Build history of the part. All positions in model axes, mm. Face numbers are marked on the shaded views. Round coordinates to 2 decimals unless told otherwise and drop trailing zeros. Loops run counter-clockwise (first coordinate to the right, second up) from the corner with the lowest first, then second, coordinate; pieces in that order, holes last.
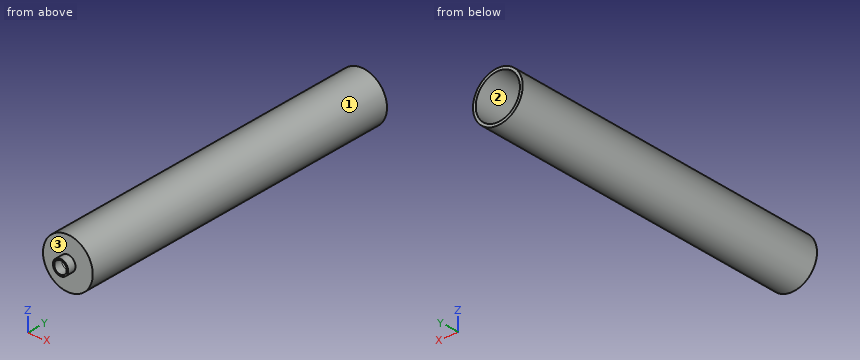
from build123d import *

# Parameters (mm, degrees)
F0_R     = 2.75
F0_R_2   = 2.25
F1_DEPTH = 3
F2_R     = 9
F3_DEPTH = 120
F4_T     = 1
F5_DEPTH = 25


# Not quite as in the source:
# - a shell that OpenCascade refuses in one call is made with other operations: the cavity is built on its own and cut out


with BuildPart() as f1:
    # F0 (on Front) → F1 (new body)
    with BuildSketch(Plane.XZ):
        Circle(F0_R)
        Circle(F0_R_2, mode=Mode.SUBTRACT)
    extrude(amount=F1_DEPTH)

    # F2 (on face) → F3 (join)
    with BuildSketch(Plane(origin=(0, 0, 0), x_dir=(-1, 0, 0), z_dir=(0, 1, 0))):
        Circle(F2_R)
    extrude(amount=F3_DEPTH)

    # F4: shell of thickness 1, made by hand


with BuildPart() as f4_core1:
    # F4_t2: copy of F1
    add(f1.part)

    # the walls: a layer under each face that stays
    f4_faces = [f4_core1.faces().sort_by_distance(p)[0] for p in [
        (9, 60, 0),
        (6, 0, -6),
        (-2.75, -1.5, 0),
        (-1.8333333333, -3, -1.8333333333),
        (-2.25, -1.5, 0),
        (0, 0, 0),
    ]]
    thicken(f4_faces, amount=-F4_T, mode=Mode.SUBTRACT)

    # F4_s3 → F4_t4 (revolve, cut)
    with BuildSketch(Plane.XY):
        Polygon((2.76, -0.01), (2.75, 1), (1.75, 1), (1.75, 0), align=None)
    revolve(axis=Axis((0, 0, 0), (0, -1, 0)), mode=Mode.SUBTRACT)

    # F4_s5 → F4_t6 (revolve, cut)
    with BuildSketch(Plane.XY):
        Polygon((2.24, -0.01), (3.25, 0), (3.25, 1), (2.25, 1), align=None)
    revolve(axis=Axis((0, 0, 0), (0, -1, 0)), mode=Mode.SUBTRACT)


with BuildPart() as f1_1:
    add(f1.part)

    # what is left inside the walls is the cavity
    f4_cavity = [f4_core1.part.solids().sort_by_distance(p)[0] for p in [
        (7.99, 80.333333, 0),
    ]]
    add(f4_cavity, mode=Mode.SUBTRACT)

    # F0 (on Front) → F5 (cut)
    with BuildSketch(Plane.XZ):
        Circle(F0_R_2)
    extrude(amount=-F5_DEPTH, mode=Mode.SUBTRACT)


solid = f1_1.part
(1) Pull direction X, two halves, no side cores. Call the marked faces 1, 2 and 3: +X half, -X half, draft (parallel to the pull), parting line (faces both ways), or undercut.
Responses:
face 1: parting line
face 2: undercut
face 3: draft
(2) Slice it at C-C on x = -6. List the corners of the cut face in (y, z), plus the area to 3 significant figures.
Responses:
outline: (0, -6.71) - (120, -6.71) - (120, -5.29) - (1, -5.29) - (1, 5.29) - (120, 5.29) - (120, 6.71) - (0, 6.71) - close
area: 351 mm2
(3) Slice it at D-D on y = 17.5. List the corners of the cut face in (x, z).
Responses:
outline: circle Ø18 at (0, 0); hole circle Ø16 at (0, 0)
(4) Slice it at A-A on x = 0. List the corners of the cut face in (y, z), plus the area to 4 significant figures.
Responses:
outline: (-3, -2.75) - (0, -2.75) - (0, -9) - (120, -9) - (120, -8) - (1, -8) - (1, -2.25) - (-3, -2.25) - close; (-3, 2.25) - (1, 2.25) - (1, 8) - (120, 8) - (120, 9) - (0, 9) - (0, 2.75) - (-3, 2.75) - close
area: 254.5 mm2
(5) Slice it at B-B on z = 0. List the corners of the cut face in (x, y), plus the area to 4 significant figures.
Responses:
outline: (-9, 0) - (-2.75, 0) - (-2.75, -3) - (-2.25, -3) - (-2.25, 1) - (-8, 1) - (-8, 120) - (-9, 120) - close; (2.25, -3) - (2.75, -3) - (2.75, 0) - (9, 0) - (9, 120) - (8, 120) - (8, 1) - (2.25, 1) - close
area: 254.5 mm2
(6) Probe line 1 (Z direction, x = 0, y = 88); line 2 (Y direction, x = 1.75, z = 7.75); line 3 (Z direction, x = 0, y = 0.5). List the from-to ranges inside material, lowest first.
Responses:
line 1: z = -9 to -8, 8 to 9
line 2: y = 0 to 1
line 3: z = -9 to -2.25, 2.25 to 9
(7) Pin check, flat tips, straight feed: P1, Ø2, axis at x = -6.5, z = -1, coming from the -Y side; P2, Ø1.5, axis at y = 105.5, z = -4.5, coming from the +X side; P3, Ø3, axis at x = 5.5, z = 2, coming from the +Y side. Stop position of each tip, or through.
Responses:
P1: stops at y = 0
P2: stops at x = 8.18
P3: stops at y = 1
